```python
from build123d import *

# Parameters (mm, degrees)
PAD_DEPTH = 15


with BuildPart() as part:
    # Sketch → Pad (new body)
    with BuildSketch(Plane.XY):
        with BuildLine():
            ThreePointArc((1.980932, -1.907461), (0, 2.75), (-1.980932, -1.907461))
            ThreePointArc((-1.925, -2.046185), (-1.939509, -1.971398), (-1.980932, -1.907461))
            Line((-1.925, -2.046185), (-1.925, -4.023292))
            ThreePointArc((-2.218407, -4.20014), (-2.021756, -4.194583), (-1.925, -4.023292))
            ThreePointArc((-3.3, 3.416504), (-4.70282, -0.667819), (-2.218407, -4.20014))
            ThreePointArc((2.474698, 5.75), (-0.639477, 5.144578), (-3.3, 3.416504))
            Line((2.474698, 5.75), (62.75, 5.75))
            Line((62.75, 2.75), (62.75, 5.75))
            Line((62.75, 2.75), (53.719164, -4.894867))
            ThreePointArc((52.75, -2.25), (51.341579, -4.266091), (53.719164, -4.894867))
            Line((52.75, 1.75), (52.75, -2.25))
            ThreePointArc((52.75, 1.75), (52.457107, 2.457107), (51.75, 2.75))
            Line((48.25, 2.75), (51.75, 2.75))
            Line((48.25, 2.75), (39.219164, -4.894867))
            ThreePointArc((38.25, -2.25), (36.841579, -4.266091), (39.219164, -4.894867))
            Line((38.25, 1.75), (38.25, -2.25))
            ThreePointArc((38.25, 1.75), (37.957107, 2.457107), (37.25, 2.75))
            Line((33.75, 2.75), (37.25, 2.75))
            Line((33.75, 2.75), (24.719164, -4.894867))
            ThreePointArc((23.75, -2.25), (22.341579, -4.266091), (24.719164, -4.894867))
            Line((23.75, 1.75), (23.75, -2.25))
            ThreePointArc((23.75, 1.75), (23.457107, 2.457107), (22.75, 2.75))
            Line((19.25, 2.75), (22.75, 2.75))
            Line((9.504324, -5.5), (19.25, 2.75))
            Line((4.925, -5.5), (9.504324, -5.5))
            Line((4.925, -5.5), (1.925, -3.046185))
            Line((1.925, -2.046185), (1.925, -3.046185))
            ThreePointArc((1.980932, -1.907461), (1.939509, -1.971398), (1.925, -2.046185))
        make_face()
    extrude(amount=PAD_DEPTH)


solid = part.part
```
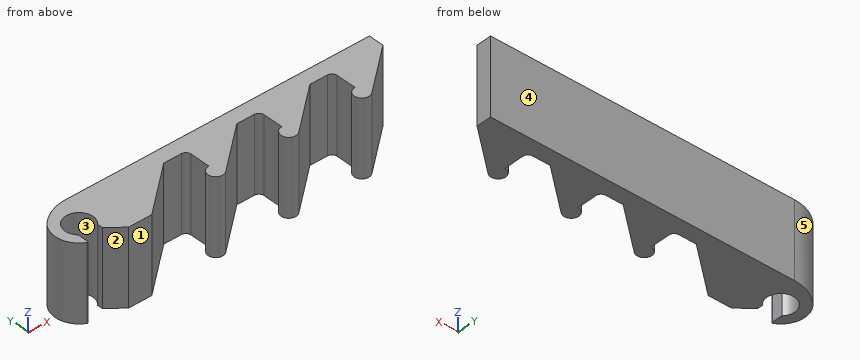
The listing builds one solid part. Answer for the finished solid, in the listing's coordinates (mm). Face numbers are marked on the shaded views. A direction names the side the tool comes from. Coordinates: 2 decimals unless noted, no trailing zeros. Loops run counter-clockwise (first coordinate to the right, second up) from the corner with the lowest first, then second, coordinate; pieces in that order, holes last. Notation, with made-up numbers: (78.25, -21.5) -> (104.25, -21.5) arc R25 cw to (104.25, -1.5) -> close; hole circle Ø2 at (12.5, 85). An arc over 180 degrees is marked (long way). Use one line per item in the form item = value. Start each with the question number.
Item 1: Flat-ended cylindrical pins translate along their axes: pin 1 Ø3 at (x, y) = (56, -3) entering from +Z; pin 2 Ø3 at (x, z) = (50, 8) entering from -Y; pin 3 Ø1.5 at (x, z) = (19.5, 12) entering from -Y; pin 4 Ø1 at (y, z) = (-3, 6) entering from +X. Find the tip coordinate at first contact, or state that the pin passes through.
Item 2: Consider L1, parallel to X at y = 0, z = 7.25; L2, parallel to X at y = -4.75, z = 12.5; L3, parallel to X at y = 1.75, z = 1.5. Determine where each line is inside the solid, lowest interval first. Write a range as [from, to].
Item 3: The part is cut by section C-C on x = 0. Determine the outline of the cut face in (y, z).
Item 4: The mould has two halves that part along X. Classify the marked faces 3, 4 and 5: released by +X, released by -X, zero draft, split by the parting line, or undercut.
Item 5: The part is cut by section D-D on x = 30.5. Determine the outline of the cut face in (y, z).
Item 6: The part is cut by section A-A on y = 0. Determine the outline of the cut face in (x, z).
Item 7: A tool of negligible diameter and unlimited length cuts with its end or side. For the marked faces 1 and 2, from which of +Z, -Z, +X, -X, +Y, -Y can it reach the whole face along a straight path? Write none if from no direction.
Answer key:
q1.pin_1 = 15
q1.pin_2 = -4.58
q1.pin_3 = 2.33
q1.pin_4 = 56.55
q2.L1 = [-4.75, -2.75], [2.75, 16], [23.75, 30.5], [38.25, 45], [52.75, 59.5]
q2.L2 = [4.01, 10.39], [22.63, 24.89], [37.13, 39.39], [51.63, 53.89]
q2.L3 = [-4.42, -2.12], [2.12, 18.07], [23.75, 32.57], [38.25, 47.07], [52.75, 61.57]
q3.outline = (2.75, 0) -> (5.37, 0) -> (5.37, 15) -> (2.75, 15) -> close
q4.face_3 = undercut
q4.face_4 = zero draft
q4.face_5 = released by -X
q5.outline = (0, 0) -> (5.75, 0) -> (5.75, 15) -> (0, 15) -> close
q6.outline = (-4.75, 0) -> (-2.75, 0) -> (-2.75, 15) -> (-4.75, 15) -> close; (2.75, 0) -> (16, 0) -> (16, 15) -> (2.75, 15) -> close; (23.75, 0) -> (30.5, 0) -> (30.5, 15) -> (23.75, 15) -> close; (38.25, 0) -> (45, 0) -> (45, 15) -> (38.25, 15) -> close; (52.75, 0) -> (59.5, 0) -> (59.5, 15) -> (52.75, 15) -> close
q7.face_1 = +Z, -Z, +X, -X, -Y
q7.face_2 = +Z, -Z, -Y
